Could you check a few things on this model? Use its own coordinates, in mm. Face numbers are marked on the shaded views. Coordinates: 2 decimals unless noted, no trailing zeros. Write each loop counter-clockwise with the first axis right and the second up, starting at its lowest first coordinate (ties: lowest second). Pieces come first, ordered by that corner, then holes. Notation, with made-up numbers: M 87,65.5 L 96,65.5 A11 ccw 96,70.5 Z; hole C -6.5,70 d9. An arc over 180 degrees is marked long. Write item = value, one per line.
```python
from build123d import *

# Parameters (mm, degrees)
F0_R     = 5
F1_DEPTH = 112
F2_R     = 7.5
F3_DEPTH = 2.5
F4_R     = 7.5
F5_DEPTH = 2.5
F7_DEPTH = 117.001
F8_R     = 0.5


with BuildPart() as f1:
    # F0 (on Right) → F1 (new body)
    with BuildSketch(Plane.YZ):
        Circle(F0_R)
    extrude(amount=F1_DEPTH)

    # F2 (on face) → F3 (join)
    with BuildSketch(Plane(origin=(0, 0, 0), x_dir=(0, -1, 0), z_dir=(-1, 0, 0))):
        Circle(F2_R)
    extrude(amount=F3_DEPTH)

    # F4 (on face) → F5 (join)
    with BuildSketch(Plane.YZ.offset(112)):
        Circle(F4_R)
    extrude(amount=F5_DEPTH)

    # F6 (on face) → F7 (cut, through all)
    with BuildSketch(Plane.YZ.offset(114.5)):
        with BuildLine():
            Line((5.5901699437, -5), (-5.5901699437, -5))
            ThreePointArc((-5.5901699437, -5), (0, -7.5), (5.5901699437, -5))
        make_face()
    extrude(amount=-F7_DEPTH, mode=Mode.SUBTRACT)

    # F8
    f8_edges = [f1.edges().sort_by_distance(p)[0] for p in [
        (-2.5, 0, -5),
        (-2.5, 0, 7.5),
        (114.5, 0, -5),
        (114.5, 0, 7.5),
        (113.25, -5.59017, -5),
        (113.25, 5.59017, -5),
        (-1.25, -5.59017, -5),
        (-1.25, 5.59017, -5),
    ]]
    fillet(f8_edges, radius=F8_R)


solid = f1.part
```
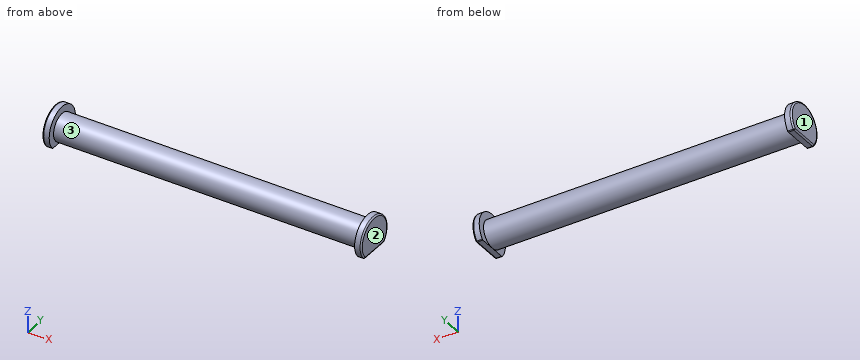
Item 1: If I drill on line 1 along X through (y, z) = (-5, 4); line 2 along Z through (x, y) = (93, -0.25); line 3 along Z through (x, y) = (31, 1.25), over which ranges is the centre line in solid material (lowest first)?
Numbers:
line_1 = -2.5 to 0, 112 to 114.5
line_2 = -4.99 to 4.99
line_3 = -4.84 to 4.84
Item 2: I'm going to push flat-ended pins straight in: P1, Ø3, axis at x = 44, z = -3, coming from the -Y side; P2, Ø6, axis at x = 58.5, z = 6, coming from the -Y side; P3, Ø3, axis at x = 50.5, z = 5.5, coming from the +Y side. Where does each tip first touch, or does it pass through?
Numbers:
P1 = -4.77
P2 = -4
P3 = 3
Item 3: Imagine slicing it at B-B (x = 81.5). Write out the boundary of the cut face in (y, z).
Numbers:
outline = C 0,0 d10
Item 4: Imagine slicing it at A-A (z = 0). Write out the boundary of the cut face in (x, y).
Numbers:
outline = M -2.5,-7 A0.5 ccw -2,-7.5 L 0,-7.5 L 0,-5 L 112,-5 L 112,-7.5 L 114,-7.5 A0.5 ccw 114.5,-7 L 114.5,7 A0.5 ccw 114,7.5 L 112,7.5 L 112,5 L 0,5 L 0,7.5 L -2,7.5 A0.5 ccw -2.5,7 Z
Item 5: If we mould it in two halves opening along X, with no side actions, what happens to the marked faces 1, 2 and 3? For each: pulls with the +X half, pulls with the -X half, needs draft (parallel to the pull), parting line crosses it, or undercut.
Numbers:
face_1 = pulls with the -X half
face_2 = pulls with the +X half
face_3 = undercut
